Part model, mm, in its own coordinate system. Round coordinates to 2 decimals unless told otherwise and drop trailing zeros. Loops run counter-clockwise (first coordinate to the right, second up) from the corner with the lowest first, then second, coordinate; pieces in that order, holes last. Notation, with made-up numbers: (17.25, 20) - (59.25, 20) arc R22 cw to (59.25, 59) - close; hole circle Ø6 at (1, 27). An arc over 180 degrees is marked (long way). Put each result on its own line as item: value.
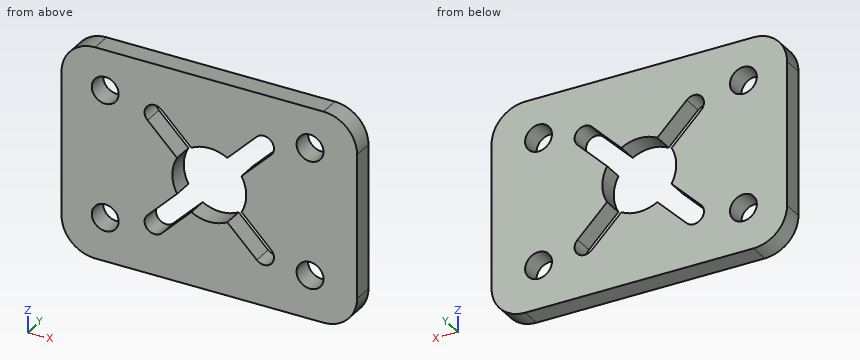
from build123d import *

# Parameters (mm, degrees)
SKETCH1_W            = 44
SKETCH1_H            = 31.5
BOSS_EXTRUDE1_DEPTH  = 3
SKETCH2_R            = 5.5
CUT_EXTRUDE1_DEPTH   = 3
CUT_EXTRUDE2_DEPTH   = 3
CUT_EXTRUDE3_DEPTH   = 3
SKETCH5_R            = 2
CUT_EXTRUDE4_DEPTH   = 3
LPATTERN1_COUNT      = 2
LPATTERN1_PITCH      = 30.5
LPATTERN1_COUNT_DIR2 = 2
LPATTERN1_PITCH_DIR2 = 19
FILLET1_R            = 5


with BuildPart() as part:
    # Sketch1 → Boss-Extrude1 (new body)
    with BuildSketch(Plane(origin=(0, 0, 0), x_dir=(1, 0, 0), z_dir=(0, 1, 0))):
        with Locations((22, 15.75)):
            Rectangle(SKETCH1_W, SKETCH1_H)
    extrude(amount=BOSS_EXTRUDE1_DEPTH)

    # Sketch2 → Cut-Extrude1 (cut)
    with BuildSketch(Plane(origin=(0, 3, 0), x_dir=(1, 0, 0), z_dir=(0, 1, 0))):
        with Locations(Location((22, 15.75, 0), (0, 0, 270))):
            Circle(SKETCH2_R)
    extrude(amount=-CUT_EXTRUDE1_DEPTH, mode=Mode.SUBTRACT)

    # Sketch3 → Cut-Extrude2 (cut)
    with BuildSketch(Plane(origin=(0, 3, 0), x_dir=(1, 0, 0), z_dir=(0, 1, 0))):
        with BuildLine():
            Line((14.928932188, 24.942388155), (31.192388155, 8.678932188))
            ThreePointArc((31.192388155, 8.678932188), (31.192388155, 6.557611845), (29.071067812, 6.557611845))
            Line((29.071067812, 6.557611845), (12.807611845, 22.821067812))
            ThreePointArc((12.807611845, 22.821067812), (12.807611845, 24.942388155), (14.928932188, 24.942388155))
        make_face()
    extrude(amount=-CUT_EXTRUDE2_DEPTH, mode=Mode.SUBTRACT)

    # Sketch4 → Cut-Extrude3 (cut)
    with BuildSketch(Plane(origin=(0, 3, 0), x_dir=(1, 0, 0), z_dir=(0, 1, 0))):
        with BuildLine():
            Line((31.192388155, 22.821067812), (14.928932188, 6.557611845))
            ThreePointArc((14.928932188, 6.557611845), (12.807611845, 6.557611845), (12.807611845, 8.678932188))
            Line((12.807611845, 8.678932188), (29.071067812, 24.942388155))
            ThreePointArc((29.071067812, 24.942388155), (31.192388155, 24.942388155), (31.192388155, 22.821067812))
        make_face()
    extrude(amount=-CUT_EXTRUDE3_DEPTH, mode=Mode.SUBTRACT)

    # Sketch5 → Cut-Extrude4 (cut)
    with BuildSketch(Plane(origin=(0, 3, 0), x_dir=(1, 0, 0), z_dir=(0, 1, 0))):
        with Locations(Location((6.5, 25, 0), (0, 0, 270))):
            Circle(SKETCH5_R)
    cut_extrude4 = extrude(amount=-CUT_EXTRUDE4_DEPTH, mode=Mode.SUBTRACT)

    # LPattern1: Cut-Extrude4 2 × 2
    with Locations(*[(i * LPATTERN1_PITCH, 0, j * LPATTERN1_PITCH_DIR2) for i in range(LPATTERN1_COUNT) for j in range(LPATTERN1_COUNT_DIR2) if (i, j) != (0, 0)]):
        add(cut_extrude4, mode=Mode.SUBTRACT)

    # Fillet1
    fillet1_edges = [part.edges().sort_by_distance(p)[0] for p in [
        (0, 1.5, -31.5),
        (44, 1.5, -31.5),
        (44, 1.5, 0),
        (0, 1.5, 0),
    ]]
    fillet(fillet1_edges, radius=FILLET1_R)


solid = part.part
1. Band-saw the part on C-C (z = -24.5). List the corners of the cut face in (x, y).
A:
outline: (0, 0) - (4.56, 0) - (4.56, 3) - (0, 3) - close; (8.44, 0) - (12.5, 0) - (12.5, 3) - (8.44, 3) - close; (15.37, 0) - (28.63, 0) - (28.63, 3) - (15.37, 3) - close; (31.5, 0) - (35.06, 0) - (35.06, 3) - (31.5, 3) - close; (38.94, 0) - (44, 0) - (44, 3) - (38.94, 3) - close
2. Band-saw the part on D-D (z = -15.5). List the corners of the cut face in (x, y), plus the area to 3 significant figures.
A:
outline: (0, 0) - (16.51, 0) - (16.51, 3) - (0, 3) - close; (27.49, 0) - (44, 0) - (44, 3) - (27.49, 3) - close
area: 99.0 mm²
3. Band-saw the part on A-A (x = 37). List the corners of the cut face in (y, z).
A:
outline: (0, -31.5) - (3, -31.5) - (3, -27) - (0, -27) - close; (0, -23) - (3, -23) - (3, -8) - (0, -8) - close; (0, -4) - (3, -4) - (3, 0) - (0, 0) - close
4. Band-saw the part on B-B (y = 0.95). List the corners of the cut face in (x, z), plus the area to 3 significant figures.
A:
outline: (0, -26.5) arc R5 ccw to (5, -31.5) - (39, -31.5) arc R5 ccw to (44, -26.5) - (44, -5) arc R5 ccw to (39, 0) - (5, 0) arc R5 ccw to (0, -5) - close; hole circle Ø4 at (6.5, -25); hole circle Ø4 at (6.5, -6); hole (12.81, -22.82) arc R1.5 ccw to (14.93, -24.94) - (19.32, -20.55) arc R5.5 ccw to (24.68, -20.55) - (29.07, -24.94) arc R1.5 ccw to (31.19, -22.82) - (26.8, -18.43) arc R5.5 ccw to (26.8, -13.07) - (31.19, -8.68) arc R1.5 ccw to (29.07, -6.56) - (24.68, -10.95) arc R5.5 ccw to (19.32, -10.95) - (14.93, -6.56) arc R1.5 ccw to (12.81, -8.68) - (17.2, -13.07) arc R5.5 ccw to (17.2, -18.43) - close; hole circle Ø4 at (37, -25); hole circle Ø4 at (37, -6)
area: 1,130 mm²
5. Probe line 1 along X through (y, z) = (2.3, -6); line 2 along X through (y, z) = (2.45, -26.5); line 3 along X through (y, z) = (2.2, -25). List the from-to ranges inside material, lowest first. Write a range as [from, to].
A:
line 1: x = [0, 4.5], [8.5, 35], [39, 44]
line 2: x = [0, 5.18], [7.82, 35.68], [38.32, 44]
line 3: x = [0, 4.5], [8.5, 12.87], [14.87, 29.13], [31.13, 35], [39, 44]
